Work out the finished part from the listing and answer in its coordinate system (mm). A direction names the side the tool comes from. Round coordinates to 2 decimals unless told otherwise and drop trailing zeros. Order: outer loops, then holes, each group sorted by start corner. A loop starts at its lowest first (then second) coordinate and runs counter-clockwise, first axis right, second up. Notation, with made-up numbers: (62.5, 27) - (85.5, 27) arc R11 cw to (85.5, 46) - close; hole circle Ø6 at (-18.5, -13). An arc over 180 degrees is marked (long way). Put each result on its own line as item: value.
Autodesk Inventor part; units mm, degrees
ref_plane "EtchPlane" through (-10, 3.25, -3.2) normal (0, 1, 0) x (1, 0, 0)
ref_plane "YZ Plane" through (0, 0, 0) normal (1, 0, 0) x (0, 1, 0)
ref_plane "XZ Plane" through (0, 0, 0) normal (0, 1, 0) x (-1, 0, 0)
sketch "LimitSwitchBody" plane through (0, 0, 0) normal (0, 0, 1) x (1, 0, 0)
  line L0 (-10, -7.65) -> (10, -7.65)
  line L1 (10, -7.65) -> (10, 7.65)
  line L2 (10, 7.65) -> (-10, 7.65)
  line L3 (-10, 7.65) -> (-10, -7.65)
  line L4 (-10, -7.65) -> (10, 7.65) construction
  line L5 (10, -7.65) -> (-10, 7.65) construction
  line L6 (-10, -0.25) -> (10, -0.25) construction
  circle A0 centre (4.85, -0.25) radius 1.15
  line L7 (3.7, -1.4) -> (6, -1.4) construction
  line L8 (6, -1.4) -> (6, 0.9) construction
  line L9 (6, 0.9) -> (3.7, 0.9) construction
  line L10 (3.7, 0.9) -> (3.7, -1.4) construction
  line L11 (3.7, -1.4) -> (6, 0.9) construction
  line L12 (6, -1.4) -> (3.7, 0.9) construction
  line L13 (0, -10.71) -> (0, 10.71) construction
  circle A1 centre (-4.85, -0.25) radius 1.15
  point P0 (0, 0)
  dimension "d0" = 20
  dimension "d1" = 15.3
  dimension "d2" = 2.3
  dimension "d3" = 4
  dimension "d4" = 7.4
extrude "LimitSwitchBodyFeature" add sketch "LimitSwitchBody" along normal mid plane 6.4
ref_plane "EtchPlane" through (-10, 3.25, -3.2) normal (0, 1, 0) x (1, 0, 0)
sketch "EtchProfile" plane through (-10, 3.25, -3.2) normal (0, 1, 0) x (1, 0, 0)
  line L0 (0, 0) -> (20, 0)
  line L1 (0, 0) -> (0, -6.4)
  line L2 (20, -6.4) -> (0, -6.4)
  line L3 (20, 0) -> (20, -6.4)
  line L4 (0.5, -5.9) -> (0.5, 0.5)
  line L5 (0.5, 0.5) -> (19.5, 0.5)
  line L6 (19.5, 0.5) -> (19.5, -5.9)
  line L7 (19.5, -5.9) -> (0.5, -5.9)
  point P0 (10, -3.2)
  dimension "d8" = 0.5
extrude "EtchFeature" cut sketch "EtchProfile" against normal blind 0.5 contours L0 L4 L7 L6 L3 L2 L1
sketch "HingeIndent" plane through (0, 0, 3.2) normal (0, 0, 1) x (1, 0, 0)
  line L0 (-10, 7.65) -> (-10, 3.25)
  line L1 (-10, 7.65) -> (-6, 7.65)
  line L2 (-6, 7.65) -> (-6, 3.65)
  line L3 (-6, 3.65) -> (-10, 3.65)
  line L4 (-10, 3.65) -> (-10, 7.65)
  circle A0 centre (-8, 5.65) radius 2
  point P0 (0, 0)
  point P1 (-8, 3.65)
  point P2 (-6, 5.65)
  dimension "d11" = 4
extrude "HingeIndentFeature" cut sketch "HingeIndent" against normal blind 0.5 contours L1 A0 L0 | A0 L3 L0 | A0 | L1 L2 A0
mirror "HingeMirrorFeature" about plane through (0, 0, 0) normal (0, 0, 1) of "HingeIndentFeature"
sketch "ButtonHousing" plane through (10, 7.65, 3.2) normal (0, 1, 0) x (1, 0, 0)
  line L0 (-24, 3.2) -> (4, 3.2) construction
  line L1 (-20, 5.9) -> (-20, 0.5) construction
  circle A0 centre (-13.6, 3.2) radius 3.2
  line L2 (0, 0) -> (-16, 0)
  point P0 (-10, 3.2)
  dimension "d14" = 6.4
extrude "ButtonHousingFeature" add sketch "ButtonHousing" along normal blind 0.5
sketch "Button" plane through (-3.6, 8.15, 0) normal (0, 1, 0) x (1, 0, 0)
  circle A0 centre (0, 0) radius 3.2 construction
  circle A1 centre (0, 0) radius 1
  point P0 (3.6, 0)
  dimension "d17" = 2
extrude "ButtonFeature" add sketch "Button" along normal blind 1
sketch "Lever" plane through (0, 0, 2.7) normal (0, 0, 1) x (1, 0, 0)
  arc A0 (-8, 3.65) -> (-6, 5.65) centre (-8, 5.65) ccw
  circle A1 centre (-8, 5.65) radius 1.75
  line L0 (-9.5155, 4.775) -> (-10.8905, 7.1566)
  line L1 (-10.8905, 7.1566) -> (-7.8595, 8.9066)
  line L2 (-7.8595, 8.9066) -> (-6.4845, 6.525)
  line L3 (-9.375, 8.0316) -> (-8, 5.65) construction
  line L4 (-10, 3.25) -> (10, 3.25)
  line L5 (-7.8595, 8.9066) -> (6.43, 17.1566)
  line L6 (-10.8905, 7.1566) -> (-11.0905, 7.503)
  line L7 (-11.0905, 7.503) -> (6.23, 17.503)
  line L8 (6.23, 17.503) -> (6.43, 17.1566)
  line L9 (-2.4303, 12.503) -> (-2.2303, 12.1566) construction
  circle A2 centre (3.3394, 19.0095) radius 1.75
  line L10 (6.23, 17.503) -> (4.855, 19.8845)
  line L11 (1.8239, 18.1345) -> (3.1989, 15.753)
  point P0 (0, 0)
  dimension "d20" = 0.25
  dimension "d21" = 2.75
  dimension "d22" = 3.5
  dimension "d23" = 120
  dimension "d24" = 20
  dimension "d25" = 0.4
extrude "LeverFeature" add sketch "Lever" along normal up to surface (0.5 mm away)
mirror "LeverMirrorFeature" about plane through (0, 0, 0) normal (0, 0, 1) of "LeverFeature"
sketch "LeverConnect" plane through (0, 0, 2.7) normal (0, 0, -1) x (-1, 0, 0)
  line L0 (10, 5.6141) -> (10, 7.65)
  line L1 (11.0905, 7.503) -> (10, 5.6141)
  line L2 (-3.1989, 15.753) -> (11.0905, 7.503)
  line L3 (-1.8239, 18.1345) -> (-3.1989, 15.753)
  arc A0 (-1.8239, 18.1345) -> (-4.855, 19.8845) centre (-3.3394, 19.0095) ccw
  line L4 (-6.43, 17.1566) -> (-4.855, 19.8845)
  line L5 (7.8595, 8.9066) -> (-6.43, 17.1566)
  line L6 (7.134, 7.65) -> (7.8595, 8.9066)
  line L7 (10, 7.65) -> (7.134, 7.65)
  point P0 (0, 0)
extrude "LeverConnectFeature" add sketch "LeverConnect" along normal up to surface (5.4 mm away)
equation "\"d26\" = d25"
properties part number "ArmLimitSwitch"
1) Given pin 1 Ø1.1 at (x, z) = (-5, 1.5) entering from +Y; pin 2 Ø1.8 at (x, y) = (-4.85, -0.25) entering from +Z; pin 3 Ø0.6 at (y, z) = (3, -1) entering from -X; pin 4 Ø2 at (y, z) = (5, -1.5) entering from -X, each flat-ended and moving along its own axis, determine where each tip first touches the part or whether it passes through.
Findings below:
pin 1: stops at y = 11.34
pin 2: passes through
pin 3: stops at x = -10
pin 4: stops at x = -10.22
2) For a pull along Y with two mould halves and no side action, classify faces 5 (the flat face through (-2.3, 12.4, -3.2)), 6 (the cylindrical face through (-3.14, 8.64, -0.89)), 7 (the flat face through (0, -7.65, 0)) as pulls with the +Y half, pulls with the -Y half, needs draft (parallel to the pull), parting line crosses it, or undercut.
Findings below:
face 5: needs draft
face 6: undercut
face 7: pulls with the -Y half
3) A cutting plane is placed at C-C on x = 7. Write down the section's boundary in (y, z), then the cut area to 3 significant figures.
Findings below:
outline: (-7.65, -3.2) - (7.65, -3.2) - (7.65, 3.2) - (3.25, 3.2) - (3.25, 2.7) - (2.75, 2.7) - (2.75, 3.2) - (-7.65, 3.2) - close
area: 97.7 mm2
4) A cutting plane is placed at B-B on x = -0.75. Write down the section's boundary in (y, z), then the cut area to 3 significant figures.
Findings below:
outline: (-7.65, -3.2) - (7.65, -3.2) - (7.65, -1.46) - (8.15, -1.46) - (8.15, 1.46) - (7.65, 1.46) - (7.65, 3.2) - (3.25, 3.2) - (3.25, 2.7) - (2.75, 2.7) - (2.75, 3.2) - (-7.65, 3.2) - close; (13.01, -3.2) - (13.47, -3.2) - (13.47, 2.7) - (13.47, 3.2) - (13.01, 3.2) - close
area: 102 mm2
5) For faces 1 (the cylindrical face through (-7.159, 4.116, -2.947)), 2 (the flat face through (-10, 4, 0)), 3 (the cylindrical face through (-6.8, 7.9, 0.1)), 4 (the flat face through (0, 2.75, 3)), determine the directions among +Z, -Z, +X, -X, +Y, -Y from which every point of the face is accessible in a straight line to the end or side of a thin tool.
Findings below:
face 1: -Z
face 2: +Z, -Z, -X, -Y
face 3: none
face 4: +Z
6) A cutting plane is placed at A-A on z = 0. Give the number of separate pieces and of enclosed holes in the cut face, then the cut area to 3 significant figures.
Findings below:
separate pieces: 1
enclosed holes: 2
area: 328 mm2
7) Straight lines are drawn through the part: L1, parallel to Y at x = 5.75, z = 3; L2, parallel to Y at x = -5.75, z = 1; L3, parallel to X at y = -0.5, z = -2.5. For each, find the intervals that lie inside material, in ascending order. Write a range as from..to.
Findings below:
L1: y = -7.65..-0.97, 0.47..2.75, 3.25..7.65, 16.76..18.33
L2: y = -7.65..-0.97, 0.47..8.15, 10.12..10.59
L3: x = -10..-5.97, -3.73..3.73, 5.97..10
8) A cutting plane is placed at D-D on y = -3.75. Write down the section's boundary in (x, z).
Findings below:
outline: (-10, -3.2) - (10, -3.2) - (10, 3.2) - (-10, 3.2) - close
